Can you work these out from the drawing? Everything is in mm from the part's minimum corner. A direction names the side the tool comes from. Round coordinates to 2 decimals unless told otherwise and drop trailing zeros. Loops run counter-clockwise (first coordinate to the right, second up) from the corner with the lowest first, then second, coordinate; pieces in that order, holes last. Notation, with made-up numbers: M 86,57 L 102,57 A8 ccw 102,68 Z; hole C 7.5,-21.5 d10. An arc over 180 degrees is marked long. Use a Markdown table: item, result.
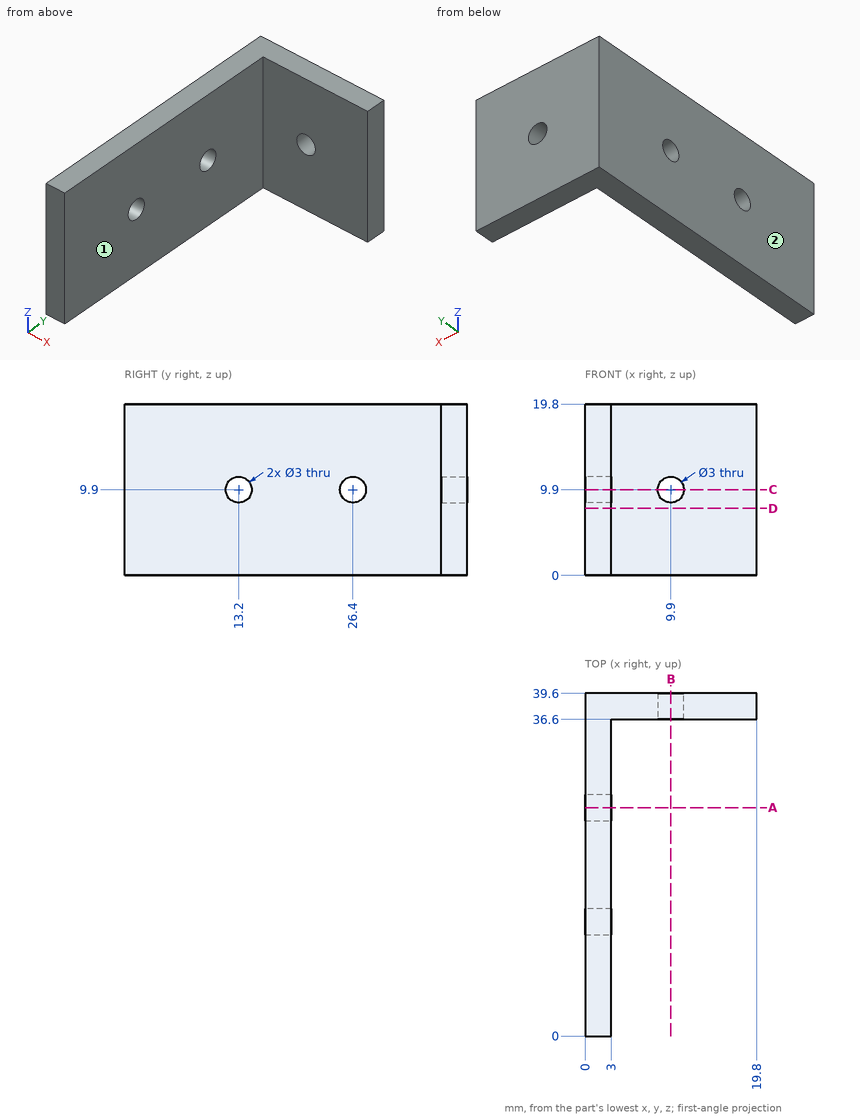
Q1. I need wall thicknesses on line 1 (Z direction, x = 0.8, y = 13.2); line 2 (X direction, y = 19, z = 18); line 3 (Y direction, x = 11.75, z = 10.5). Which ranges of each line are inside material? Lowest first, please. Write a range as from..to.
Return value:
| item | result |
|---|---|
| line 1 | z = 0..8.4, 11.4..19.8 |
| line 2 | x = 0..3 |
| line 3 | y = 36.6..39.6 |
Q2. Imagine slicing it at B-B, the plane x = 9.9. Please give me the cut outline in (y, z).
Return value:
| item | result |
|---|---|
| outline | M 36.6,0 L 39.6,0 L 39.6,8.4 L 36.6,8.4 Z; M 36.6,11.4 L 39.6,11.4 L 39.6,19.8 L 36.6,19.8 Z |
Q3. Imagine slicing it at C-C, the plane z = 9.9. Please give me the cut outline in (x, y).
Return value:
| item | result |
|---|---|
| outline | M 0,0 L 3,0 L 3,11.7 L 0,11.7 Z; M 0,14.7 L 3,14.7 L 3,24.9 L 0,24.9 Z; M 0,27.9 L 3,27.9 L 3,36.6 L 8.4,36.6 L 8.4,39.6 L 0,39.6 Z; M 11.4,36.6 L 19.8,36.6 L 19.8,39.6 L 11.4,39.6 Z |
Q4. Imagine slicing it at D-D, the plane z = 7.75. Please give me the cut outline in (x, y), then the cut area to 3 significant figures.
Return value:
| item | result |
|---|---|
| outline | M 0,0 L 3,0 L 3,36.6 L 19.8,36.6 L 19.8,39.6 L 0,39.6 Z |
| area | 169 mm^2 |
Q5. Imagine slicing it at A-A, the plane y = 26.4. Please give me the cut outline in (x, z).
Return value:
| item | result |
|---|---|
| outline | M 0,0 L 3,0 L 3,8.4 L 0,8.4 Z; M 0,11.4 L 3,11.4 L 3,19.8 L 0,19.8 Z |
Q6. For the marked faces 1 and 2, which set-ups out of +Z, -Z, +X, -X, +Y, -Y let a thin tool reach every point of the face, with its end or its side?
Return value:
| item | result |
|---|---|
| face 1 | +Z, -Z, +X, -Y |
| face 2 | +Z, -Z, -X, +Y, -Y |
Q7. Will these pins go through, and if not, where does the flat tip stop? P1, Ø6, axis at y = 9.5, z = 6.5, coming from the +X side; P2, Ø3, axis at x = 3, z = 2.5, coming from the -Y side.
Return value:
| item | result |
|---|---|
| P1 | stops at x = 3 |
| P2 | stops at y = 0 |
